from build123d import *

# Parameters (mm, degrees)
F1_DEPTH    = 20
F2_T1_DEPTH = 20
F2_T3_DEPTH = 401
F3_W        = 414
F3_H        = 462.4
F4_DEPTH    = 25.4
F5_T1_DEPTH = 20


# Not quite as in the source:
# - a fillet or chamfer that OpenCascade refuses, or shapes differently, is made with other operations: its cross-section is extruded or revolved along the edge and cut away or added


with BuildPart() as f1:
    # F0 (on Front) → F1 (new body)
    with BuildSketch(Plane.XZ):
        Polygon((293.8, 477), (-293.8, 477), (-293.8, -72.2), (-120.2, -72.2), (-120.2, -332.6), (120.2, -332.6), (120.2, -72.2), (293.8, -72.2), align=None)
    extrude(amount=F1_DEPTH)

    # F2: fillet of radius 76.2 on 6 edges, made by hand

    # F2_s2 → F2_t1 (join)
    with BuildSketch(Plane.XZ):
        with BuildLine():
            add(Edge.make_bspline(
                [(-196.4, -72.2), (-120.2, -72.2), (-120.2, -148.4)],
                knots=[0, 0, 0, 1, 1, 1], degree=2, weights=[1, 1, 1]))
            Line((-120.2, -148.4), (-120.2, -72.2))
            Line((-120.2, -72.2), (-196.4, -72.2))
        make_face()
        with BuildLine():
            add(Edge.make_bspline(
                [(120.2, -148.4), (120.2, -72.2), (196.4, -72.2)],
                knots=[0, 0, 0, 1, 1, 1], degree=2, weights=[1, 1, 1]))
            Line((196.4, -72.2), (120.2, -72.2))
            Line((120.2, -72.2), (120.2, -148.4))
        make_face()
    extrude(amount=F2_T1_DEPTH)

    # F2_s4 → F2_t3 (cut)
    with BuildSketch(Plane.XZ.offset(-190.5)):
        with BuildLine():
            add(Edge.make_bspline(
                [(-293.8, 4), (-293.8, -72.2), (-217.6, -72.2)],
                knots=[0, 0, 0, 1, 1, 1], degree=2, weights=[1, 1, 1]))
            Line((-217.6, -72.2), (-293.8, -72.2))
            Line((-293.8, -72.2), (-293.8, 4))
        make_face()
        with BuildLine():
            add(Edge.make_bspline(
                [(44, -332.6), (120.2, -332.6), (120.2, -256.4)],
                knots=[0, 0, 0, 1, 1, 1], degree=2, weights=[1, 1, 1]))
            Line((120.2, -256.4), (120.2, -332.6))
            Line((120.2, -332.6), (44, -332.6))
        make_face()
        with BuildLine():
            add(Edge.make_bspline(
                [(293.8, 4), (293.8, -72.2), (217.6, -72.2)],
                knots=[0, 0, 0, 1, 1, 1], degree=2, weights=[1, 1, 1]))
            Line((217.6, -72.2), (293.8, -72.2))
            Line((293.8, -72.2), (293.8, 4))
        make_face()
        with BuildLine():
            add(Edge.make_bspline(
                [(-120.2, -256.4), (-120.2, -332.6), (-44, -332.6)],
                knots=[0, 0, 0, 1, 1, 1], degree=2, weights=[1, 1, 1]))
            Line((-44, -332.6), (-120.2, -332.6))
            Line((-120.2, -332.6), (-120.2, -256.4))
        make_face()
    extrude(amount=F2_T3_DEPTH, mode=Mode.SUBTRACT)

    # F3 (on Front) → F4 (cut)
    with BuildSketch(Plane.XZ):
        with Locations((0, 202.4)):
            Rectangle(F3_W, F3_H)
    extrude(amount=F4_DEPTH, mode=Mode.SUBTRACT)

    # F5: fillet of radius 76.2 on 2 edges, made by hand

    # F5_s2 → F5_t1 (join)
    with BuildSketch(Plane.XZ):
        with BuildLine():
            add(Edge.make_bspline(
                [(-130.8, 433.6), (-207, 433.6), (-207, 357.4)],
                knots=[0, 0, 0, 1, 1, 1], degree=2, weights=[1, 1, 1]))
            Line((-207, 357.4), (-207, 433.6))
            Line((-207, 433.6), (-130.8, 433.6))
        make_face()
        with BuildLine():
            add(Edge.make_bspline(
                [(207, 357.4), (207, 433.6), (130.8, 433.6)],
                knots=[0, 0, 0, 1, 1, 1], degree=2, weights=[1, 1, 1]))
            Line((130.8, 433.6), (207, 433.6))
            Line((207, 433.6), (207, 357.4))
        make_face()
    extrude(amount=F5_T1_DEPTH)


solid = f1.part
Geometry check sheet. Reference: the model listing, model coordinates, mm. A direction names the side the tool comes from. Give positions to 0.01 mm unless a question says otherwise; leave off trailing zeros. Loops run counter-clockwise (first coordinate to the right, second up) from the corner with the lowest first, then second, coordinate; pieces in that order, holes last.
(1) Set-up check for faces 5 (the flat face through (207, -10, -72.2)), 6 (the flat face through (-120.2, -10, -202)), 7 (the flat face through (-2, -10, 433.6)), 8 (the flat face through (293.8, -10, 237)): record each of +Z, -Z, +X, -X, +Y, -Y from which the full face is reachable in a straight line by a thin tool's end or side.
From the geometry:
face 5: -Z, +X, +Y, -Y
face 6: -Z, -X, +Y, -Y
face 7: +Y, -Y
face 8: +Z, -Z, +X, +Y, -Y
(2) Release check for a two-part mould opening along Z. For faces 1 (the flat face through (-207, -10, -72.2)), 2 (the flat face through (207, -10, 162)), 3 (the flat face through (-207, -10, 162)), 4 (the flat face through (-42, 0, -46)) record: released by +Z, released by -Z, zero draft, split by the parting line, or undercut.
From the geometry:
face 1: released by -Z
face 2: undercut
face 3: undercut
face 4: zero draft
(3) Depth check by flat-ended pin: pin 1 Ø8 at (x, y) = (-216, -14) entering from -Z; pin 2 Ø2 at (x, y) = (-65.5, -14.5) entering from -Z; pin 3 Ø6 at (y, z) = (-9, -224) entering from +X. Enter the tip coordinate at first touch or a pass-through.
From the geometry:
pin 1: stops at z = -72.2
pin 2: stops at z = -331
pin 3: stops at x = 120.2
(4) Section check B-B on z = -218.5. Record the cut outline in (x, y).
From the geometry:
outline: (-120.2, -20) - (120.2, -20) - (120.2, 0) - (-120.2, 0) - close
(5) Section check A-A on z = 196. Record the cut outline in (x, y).
From the geometry:
outline: (-293.8, -20) - (-207, -20) - (-207, 0) - (-293.8, 0) - close; (207, -20) - (293.8, -20) - (293.8, 0) - (207, 0) - close
(6) Thickness scan on L1, parallel to Z at x = 30.5, y = -2.5; L2, parallel to X at y = -15.75, z = 242.5; L3, parallel to X at y = -14, z = 362. Record the ranges inside material, lowest first.
From the geometry:
L1: z = -332.6 to -28.8, 433.6 to 477
L2: x = -293.8 to -207, 207 to 293.8
L3: x = -293.8 to -206.93, 206.93 to 293.8
